```python
from build123d import *

# Parameters (mm, degrees)
F0_W     = 279.4
F0_H     = 635
F1_DEPTH = 374.65
F2_DEPTH = 6.35


# Not quite as in the source:
# - a feature names something its author has since deleted; it is built from what else it names


with BuildPart() as f1:
    # F0 (on Front) → F1 (new body)
    with BuildSketch(Plane.XZ):
        Polygon((263.9267770052, 0), (289.3267770052, 0), (289.3267770052, 762), (263.9267770052, 762), (-117.0732229948, 762), (-117.0732229948, 0), align=None)
        with Locations((86.1267770052, 381)):
            Rectangle(F0_W, F0_H, mode=Mode.SUBTRACT)
        with Locations((86.1267770052, 381)):
            Rectangle(F0_W, F0_H)
    extrude(amount=-F1_DEPTH)

    # F0 (on Front) → F2 (cut)
    with BuildSketch(Plane.XZ):
        with Locations((86.1267770052, 381)):
            Rectangle(F0_W, F0_H)
    extrude(amount=-F2_DEPTH, mode=Mode.SUBTRACT)


solid = f1.part
```
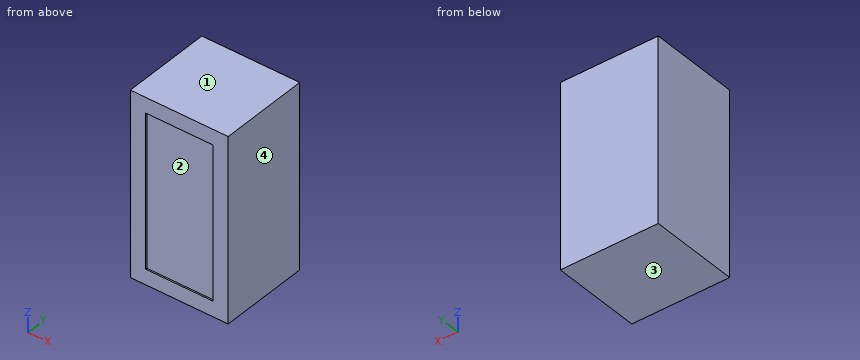
Can you work these out from the model? Positions are in its coordinate system, mm. Face numbers are marked on the shaded views. Coordinates: 2 decimals unless noted, no trailing zeros. Put each result on its own line as item: value. Start each with the question number.
Q1. If I drill on line 1 (Y direction, x = 61, z = 72), over which ranges is the centre line in solid material (lowest first)? Write a range as [from, to].
Q2. I'm going to push a flat-ended pin straight in: P1, Ø3, axis at x = -1, z = 448, coming from the -Y side. Where does the tip first touch, or does it pass through?
Q3. Thinking about a two-plate mould opening in Z: for the marked faces 1, 2, 3 and 4, which applies, pulls with the +Z half, pulls with the -Z half, needs draft (parallel to the pull), parting line crosses it, or undercut?
Taken from the geometry:
1. line 1: y = [6.35, 374.65]
2. P1: stops at y = 6.35
3. face 1: pulls with the +Z half
3. face 2: undercut
3. face 3: pulls with the -Z half
3. face 4: needs draft
